```python
from build123d import *

# Parameters (mm, degrees)
ESQUISSE1_W             = 28.5
ESQUISSE1_H             = 46.5
BOSS_EXTRU_1_DEPTH      = 34
ESQUISSE2_R             = 9.75
ESQUISSE2_R_2           = 0.8
BOSS_EXTRU_2_DEPTH      = 2
ESQUISSE3_R             = 1.025
ENL_V_MAT_EXTRU_1_DEPTH = 3
ESQUISSE4_R             = 1.025
ENL_V_MAT_EXTRU_2_DEPTH = 3
ENL_V_START             = -3
ESQUISSE5_R             = 1.025
ENL_V_MAT_EXTRU_3_DEPTH = 3
ESQUISSE6_R             = 1.025
ENL_V_MAT_EXTRU_4_DEPTH = 3
CHANFREIN1_SIZE         = 2


with BuildPart() as part:
    # Esquisse1 → Boss.-Extru.1 (new body)
    with BuildSketch(Plane.XY):
        Rectangle(ESQUISSE1_W, ESQUISSE1_H)
    extrude(amount=BOSS_EXTRU_1_DEPTH)

    # Esquisse2 → Boss.-Extru.2 (add)
    with BuildSketch(Plane.XY.offset(34)):
        with Locations((0, 12)):
            Circle(ESQUISSE2_R)
        with Locations((0, 20)):
            Circle(ESQUISSE2_R_2, mode=Mode.SUBTRACT)
        with Locations((5.656854249, 17.656854249)):
            Circle(ESQUISSE2_R_2, mode=Mode.SUBTRACT)
        with Locations((8, 12)):
            Circle(ESQUISSE2_R_2, mode=Mode.SUBTRACT)
        with Locations((5.656854249, 6.343145751)):
            Circle(ESQUISSE2_R_2, mode=Mode.SUBTRACT)
        with Locations((0, 4)):
            Circle(ESQUISSE2_R_2, mode=Mode.SUBTRACT)
        with Locations((-5.656854249, 6.343145751)):
            Circle(ESQUISSE2_R_2, mode=Mode.SUBTRACT)
        with Locations((-8, 12)):
            Circle(ESQUISSE2_R_2, mode=Mode.SUBTRACT)
        with Locations((-5.656854249, 17.656854249)):
            Circle(ESQUISSE2_R_2, mode=Mode.SUBTRACT)
    extrude(amount=BOSS_EXTRU_2_DEPTH)

    # Esquisse3 → Enlèv. mat.-Extru.1 (cut)
    with BuildSketch(Plane(origin=(0, 23.25, 0), x_dir=(1, 0, 0), z_dir=(0, 1, 0))):
        with Locations(Location((-8, -23, 0), (0, 0, 270))):
            Circle(ESQUISSE3_R)
        with Locations(Location((8, -23, 0), (0, 0, 270))):
            Circle(ESQUISSE3_R)
    extrude(amount=-ENL_V_MAT_EXTRU_1_DEPTH, mode=Mode.SUBTRACT)

    # Esquisse4 → Enlèv. mat.-Extru.2 (cut)
    with BuildSketch(Plane.ZY.offset(14.25)):
        with Locations(Location((23, 8, 0), (0, 0, 270))):
            Circle(ESQUISSE4_R)
        with Locations(Location((11, 8, 0), (0, 0, 270))):
            Circle(ESQUISSE4_R)
        with Locations(Location((23, -16, 0), (0, 0, 270))):
            Circle(ESQUISSE4_R)
        with Locations(Location((11, -16, 0), (0, 0, 270))):
            Circle(ESQUISSE4_R)
    extrude(amount=-ENL_V_MAT_EXTRU_2_DEPTH, mode=Mode.SUBTRACT)

    # Esquisse5 → Enlèv. mat.-Extru.3 (cut)
    with BuildSketch(Plane(origin=(14.25, 0, 0), x_dir=(0, 0, -1), z_dir=(1, 0, 0)).offset(ENL_V_START)):
        with Locations(Location((-11, -16, 0), (0, 0, 270))):
            Circle(ESQUISSE5_R)
        with Locations(Location((-23, -16, 0), (0, 0, 270))):
            Circle(ESQUISSE5_R)
        with Locations(Location((-23, 8, 0), (0, 0, 270))):
            Circle(ESQUISSE5_R)
        with Locations(Location((-11, 8, 0), (0, 0, 270))):
            Circle(ESQUISSE5_R)
    extrude(amount=ENL_V_MAT_EXTRU_3_DEPTH, mode=Mode.SUBTRACT)

    # Esquisse6 → Enlèv. mat.-Extru.4 (cut)
    with BuildSketch(Plane.XZ.offset(23.25).offset(ENL_V_START)):
        with Locations(Location((-8, 23, 0), (0, 0, 90))):
            Circle(ESQUISSE6_R)
        with Locations(Location((8, 23, 0), (0, 0, 90))):
            Circle(ESQUISSE6_R)
        with Locations(Location((-8, 11, 0), (0, 0, 270))):
            Circle(ESQUISSE6_R)
        with Locations(Location((8, 11, 0), (0, 0, 270))):
            Circle(ESQUISSE6_R)
    extrude(amount=ENL_V_MAT_EXTRU_4_DEPTH, mode=Mode.SUBTRACT)

    # Chanfrein1
    chanfrein1_edges = [part.edges().sort_by_distance(p)[0] for p in [
        (-14.25, 23.25, 17),
        (14.25, 23.25, 17),
        (14.25, -23.25, 17),
        (-14.25, -23.25, 17),
    ]]
    chamfer(chanfrein1_edges, length=CHANFREIN1_SIZE)


solid = part.part
```
The listing builds one solid part. Answer for the finished solid, in the listing's coordinates (mm). A direction names the side the tool comes from. Give positions to 0.01 mm unless a question says otherwise; leave off trailing zeros. Order: outer loops, then holes, each group sorted by start corner. A loop starts at its lowest first (then second) coordinate and runs counter-clockwise, first axis right, second up. Notation, with made-up numbers: (-5.75, -10) -> (31.25, -10) arc R28 cw to (31.25, 14) -> close; hole circle Ø8 at (-15, 28.25). An arc over 180 degrees is marked (long way). Write each question's results on one line, items separated by ' | '.
Q1. Determine the mould class of faces 1 (the face through (11.25, 8, 23)), 2 (the face through (13.3, -22.2, 16.8)), 3 (the face through (8, 20.25, 23)) for opening direction Y: pulls with the +Y half, pulls with the -Y half, needs draft (parallel to the pull), parting line crosses it, or undercut.
Checked values:
face 1: undercut | face 2: pulls with the -Y half | face 3: pulls with the +Y half
Q2. The part is cut by section C-C, the plane x = 1.75. Give the vertices of the cut face in (y, z).
Checked values:
outline: (-23.25, 0) -> (23.25, 0) -> (23.25, 34) -> (21.59, 34) -> (21.59, 36) -> (2.41, 36) -> (2.41, 34) -> (-23.25, 34) -> close
Q3. Straight lines are drawn through the part: probe 1 along Z at (x, y) = (-13.2, -16) (3 decimals); probe 2 along X at (y, z) = (-21.2, 11) (3 decimals); probe 3 along Y at (x, z) = (12.7, 23) (3 decimals). For each, find the intervals that lie inside material, in ascending order. Write a range as from..to.
Checked values:
probe 1: z = 0..9.975, 12.025..21.975, 24.025..34 | probe 2: x = -14.25..-9.025, -6.975..6.975, 9.025..14.25 | probe 3: y = -22.8..-17.025, -14.975..6.975, 9.025..22.8
Q4. The part is cut by section B-B, the plane y = 12. Give the vertices of the cut face in (x, z).
Checked values:
outline: (-14.25, 0) -> (14.25, 0) -> (14.25, 34) -> (9.75, 34) -> (9.75, 36) -> (8.8, 36) -> (8.8, 34) -> (7.2, 34) -> (7.2, 36) -> (-7.2, 36) -> (-7.2, 34) -> (-8.8, 34) -> (-8.8, 36) -> (-9.75, 36) -> (-9.75, 34) -> (-14.25, 34) -> close
Q5. The part is cut by section D-D, the plane x = 8. Give the vertices of the cut face in (y, z) (3 decimals).
Checked values:
outline: (-23.25, 0) -> (23.25, 0) -> (23.25, 21.975) -> (20.25, 21.975) -> (20.25, 24.025) -> (23.25, 24.025) -> (23.25, 34) -> (17.573, 34) -> (17.573, 36) -> (12.8, 36) -> (12.8, 34) -> (11.2, 34) -> (11.2, 36) -> (6.427, 36) -> (6.427, 34) -> (-23.25, 34) -> (-23.25, 24.025) -> (-20.25, 24.025) -> (-20.25, 21.975) -> (-23.25, 21.975) -> (-23.25, 12.025) -> (-20.25, 12.025) -> (-20.25, 9.975) -> (-23.25, 9.975) -> close
Q6. Each of these flat-tipped pins is pushed along its axis until it touches: P1, Ø0.5, axis at x = 8, y = 12, coming from the +Z side; P2, Ø1.2, axis at y = 8, z = 23, coming from the +X side; P3, Ø0.6, axis at y = -16, z = 23, coming from the -X side. Where does it stop, or does it pass through?
Checked values:
P1: stops at z = 34 | P2: stops at x = 11.25 | P3: stops at x = -11.25
Q7. Which of the six approach directions +Z, -Z, +X, -X, +Y, -Y give full straight-line access (tool end or side, diameter ignored) to faces 4 (the face through (-8, -20.25, 11)), 5 (the face through (-11.25, -16, 23)), 6 (the face through (12.73, 8.76, 10.31)), 7 (the face through (7.2, 12, 35))?
Checked values:
face 4: -Y | face 5: -X | face 6: +X | face 7: +Z
